from build123d import *

# Parameters (mm, degrees)
ESQUISSE1_R        = 1.75
ESQUISSE1_W        = 27
ESQUISSE1_H        = 43
BOSS_EXTRU_1_DEPTH = 6
CONG_1_R           = 3.5


with BuildPart() as part:
    # Esquisse1 → Boss.-Extru.1 (new body)
    with BuildSketch(Plane.XY):
        with BuildLine():
            Line((109.450836441, 80), (-109.450836441, 80))
            ThreePointArc((-109.450836441, 80), (-116.203114748, 77.203114748), (-119, 70.450836441))
            Line((-119, 70.450836441), (-119, -70.450836441))
            ThreePointArc((-119, -70.450836441), (-116.203114748, -77.203114748), (-109.450836441, -80))
            Line((-109.450836441, -80), (109.450836441, -80))
            ThreePointArc((109.450836441, -80), (116.203114748, -77.203114748), (119, -70.450836441))
            Line((119, -70.450836441), (119, 70.450836441))
            ThreePointArc((119, 70.450836441), (116.203114748, 77.203114748), (109.450836441, 80))
        make_face()
        with Locations((109, -70)):
            Circle(ESQUISSE1_R, mode=Mode.SUBTRACT)
        with Locations((109, 70)):
            Circle(ESQUISSE1_R, mode=Mode.SUBTRACT)
        with Locations((-24, 27)):
            Circle(ESQUISSE1_R, mode=Mode.SUBTRACT)
        with Locations((-24, 70)):
            Circle(ESQUISSE1_R, mode=Mode.SUBTRACT)
        with Locations((109, 27)):
            Circle(ESQUISSE1_R, mode=Mode.SUBTRACT)
        with Locations((109, -24.5)):
            Circle(ESQUISSE1_R, mode=Mode.SUBTRACT)
        with Locations((-112, -24.5)):
            Circle(ESQUISSE1_R, mode=Mode.SUBTRACT)
        with Locations((84, 75)):
            Circle(ESQUISSE1_R, mode=Mode.SUBTRACT)
        with Locations((84, -75)):
            Circle(ESQUISSE1_R, mode=Mode.SUBTRACT)
        with Locations((-109, -70)):
            Circle(ESQUISSE1_R, mode=Mode.SUBTRACT)
        with Locations((-109, 70)):
            Circle(ESQUISSE1_R, mode=Mode.SUBTRACT)
        with Locations((-84, -75)):
            Circle(ESQUISSE1_R, mode=Mode.SUBTRACT)
        with Locations((-84, 75)):
            Circle(ESQUISSE1_R, mode=Mode.SUBTRACT)
        with Locations((0, 35)):
            Circle(ESQUISSE1_R, mode=Mode.SUBTRACT)
        with Locations((0, -34.75)):
            Circle(ESQUISSE1_R, mode=Mode.SUBTRACT)
        with Locations((-12.5, 29.75)):
            Circle(ESQUISSE1_R, mode=Mode.SUBTRACT)
        with Locations((12.5, 29.75)):
            Circle(ESQUISSE1_R, mode=Mode.SUBTRACT)
        with Locations((12.5, -29.75)):
            Circle(ESQUISSE1_R, mode=Mode.SUBTRACT)
        with Locations((-12.5, -29.75)):
            Circle(ESQUISSE1_R, mode=Mode.SUBTRACT)
        with Locations((-66.5, 55)):
            Circle(ESQUISSE1_R, mode=Mode.SUBTRACT)
        with Locations((-66.5, -5.5)):
            Circle(ESQUISSE1_R, mode=Mode.SUBTRACT)
        with Locations((-58, -70.9)):
            Circle(ESQUISSE1_R, mode=Mode.SUBTRACT)
        with Locations((55, -70.9)):
            Circle(ESQUISSE1_R, mode=Mode.SUBTRACT)
        Rectangle(ESQUISSE1_W, ESQUISSE1_H, mode=Mode.SUBTRACT)
        with BuildLine():
            Line((99, -10), (74, -10))
            ThreePointArc((74, -10), (64, 0), (74, 10))
            Line((74, 10), (99, 10))
            ThreePointArc((99, 10), (109, 0), (99, -10))
        make_face(mode=Mode.SUBTRACT)
    extrude(amount=BOSS_EXTRU_1_DEPTH)

    # Congé1
    cong_1_edges = [part.edges().sort_by_distance(p)[0] for p in [
        (13.5, 21.5, 3),
        (-13.5, 21.5, 3),
        (-13.5, -21.5, 3),
        (13.5, -21.5, 3),
    ]]
    fillet(cong_1_edges, radius=CONG_1_R)


solid = part.part
Source: CAD feature listing. Evaluate the final solid. Frame: model axes, mm. A direction names the side the tool comes from. Give positions to 0.01 mm unless a question says otherwise; leave off trailing zeros. Write each loop counter-clockwise with the first axis right and the second up, starting at its lowest first coordinate (ties: lowest second). Pieces come first, ordered by that corner, then holes. Notation, with made-up numbers: M 11.25,47.25 L 31.25,47.25 A29 cw 31.25,80.25 Z; hole C -3,61 d8. An arc over 180 degrees is marked long. Return JSON: item names as keys, results as strings. Group by question number.
1) Cut plane B-B, the plane z = 3.85. Give the number of separate pieces and of enclosed holes in the cut face, plus the area to 3 significant figures.
2) Cut plane A-A, the plane x = 66.5. Output: boundary loops of the cut face in (y, z).
3) Pull-direction query (Y, two-part tool) for faces 3 (the face through (119, -1, 3)), 4 (the face through (2, 80, 3)), 5 (the face through (-116.277, -77.128, 2.958)), 6 (the face through (86, 10, 3)); classes: pulls with the +Y half, pulls with the -Y half, needs draft (parallel to the pull), parting line crosses it, or undercut.
4) Pin query (flat end, axial travel): P1, Ø3, axis at x = -12.5, y = 29.75, coming from the +Z side. Return the tip coordinate at first contact, or that it passes through.
5) Material intervals for line 1 along Y through (x, z) = (0, 3.75); line 2 along Y through (x, z) = (84, 2.85); line 3 along X through (y, z) = (70, 2.05), sorted ascending. Write a range as [from, to].
6) Set-up query: faces 1 (the face through (-28, 1, 0)), 2 (the face through (-13.5, 0, 3)). Return all of +Z, -Z, +X, -X, +Y, -Y with unobstructed straight access to the full face (end or side cutting, diameter ignored); none if empty.
Recorded:
{
 "1": {"separate pieces": "1", "enclosed holes": "25", "area": "35,800 mm²"},
 "2": {"outline": "M -80,0 L -6.61,0 L -6.61,6 L -80,6 Z; M 6.61,0 L 80,0 L 80,6 L 6.61,6 Z"},
 "3": {"face 3": "needs draft", "face 4": "pulls with the +Y half", "face 5": "pulls with the -Y half", "face 6": "undercut"},
 "4": {"P1": "passes through"},
 "5": {"line 1": "y = [-80, -36.5], [-33, -21.5], [21.5, 33.25], [36.75, 80]", "line 2": "y = [-80, -76.75], [-73.25, -10], [10, 73.25], [76.75, 80]", "line 3": "x = [-119, -110.75], [-107.25, -25.75], [-22.25, 107.25], [110.75, 119]"},
 "6": {"face 1": "-Z, +X, -X, +Y, -Y", "face 2": "+Z, -Z"}
}
